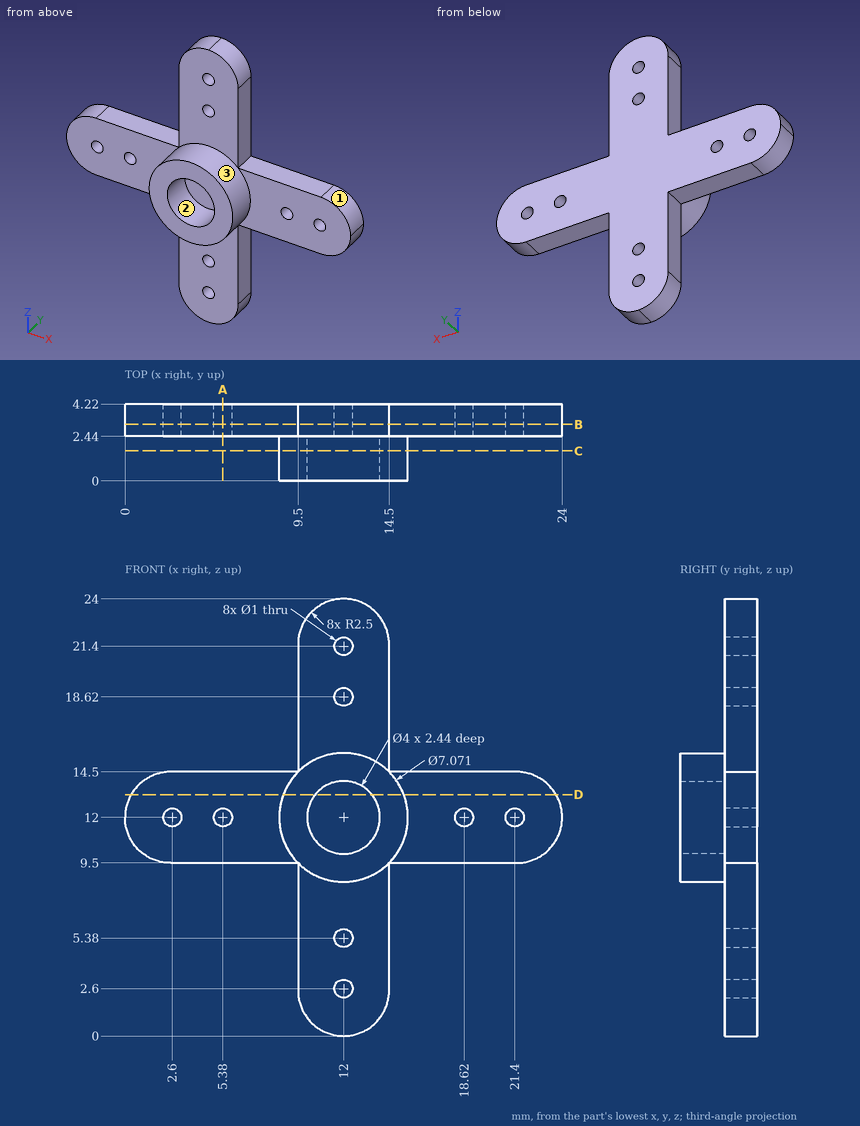
Geometry check sheet. Reference: drawing and pictorial views, mm from the part's lowest x, y, z. Round coordinates to 2 decimals unless told otherwise and drop trailing zeros. Order: outer loops, then holes, each group sorted by start corner. A loop starts at its lowest first (then second) coordinate and runs counter-clockwise, first axis right, second up. Notation, with made-up numbers: M 77.25,5.25 L 120.25,5.25 A31 ccw 120.25,30.25 Z; hole C 5.25,-36 d11. An arc over 180 degrees is marked long. One line per item, written item: value. Start each with the question number.
1. Release check for a two-part mould opening along X. For the marked faces 1, 2 and 3 record: released by +X, released by -X, zero draft, split by the parting line, or undercut.
2. Scan lines: line 1 along X through (y, z) = (2.85, 21.4); line 2 along Z through (x, y) = (8.75, 3.7); line 3 along X through (y, z) = (1.85, 12). Record each from-to range of solid material in increasing order.
3. Section check D-D on z = 13.25. Enter the section's corners in (x, y) (3 decimals).
4. Section check A-A on x = 5.38. Enter the section's corners in (y, z).
5. Gauge pin test, flat ends, axial feed: P1, Ø0.5, axis at y = 3.5, z = 17.5, coming from the -X side; P2, Ø1.5, axis at y = 0.5, z = 14, coming from the -X side; P3, Ø0.9, axis at y = 3, z = 5.5, coming from the +X side. Record the tip position at first contact, or that the pin passes through.
6. Section check B-B on y = 3.1. Give the number of separate pieces and of enclosed holes in the cut face, and give its area (3 significant figures).
7. Section check C-C on y = 1.65. Enter the section's corners in (x, z), and give its area (3 significant figures).
Results found:
1. face 1: released by +X
1. face 2: undercut
1. face 3: split by the parting line
2. line 1: 9.5 to 11.5, 12.5 to 14.5
2. line 2: 9.5 to 14.5
2. line 3: 8.46 to 10, 14 to 15.54
3. outline: M 0.335,2.44 L 8.693,2.44 L 8.693,0 L 10.439,0 L 10.439,2.44 L 13.561,2.44 L 13.561,0 L 15.307,0 L 15.307,2.44 L 23.665,2.44 L 23.665,4.22 L 0.335,4.22 Z
4. outline: M 2.44,9.5 L 4.22,9.5 L 4.22,11.5 L 2.44,11.5 Z; M 2.44,12.5 L 4.22,12.5 L 4.22,14.5 L 2.44,14.5 Z
5. P1: x = 9.5
5. P2: x = 8.69
5. P3: x = 14.5
6. separate pieces: 1
6. enclosed holes: 8
6. area: 198 mm^2
7. outline: C 12,12 d7.07; hole C 12,12 d4
7. area: 26.7 mm^2
